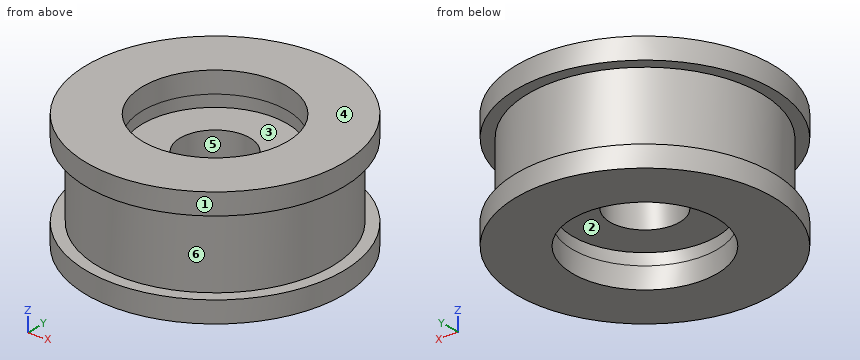
Autodesk Inventor part; units mm, degrees
ref_plane "Work Plane1" through (0, 0, 25) normal (0, 0, 1) x (1, 0, 0)
ref_plane "YZ Plane" through (0, 0, 0) normal (1, 0, 0) x (0, 1, 0)
ref_plane "XZ Plane" through (0, 0, 0) normal (0, 1, 0) x (-1, 0, 0)
sketch "Sketch1" plane through (0, 0, 0) normal (0, 0, 1) x (1, 0, 0)
  circle A0 centre (0, 0) radius 31
  circle A1 centre (0, 0) radius 55
  dimension "d0" = 62
  dimension "d1" = 110
extrude "Extrusion1" add sketch "Sketch1" along normal blind 9.12
sketch "Sketch2" plane through (0, 0, 9.12) normal (0, 0, 1) x (1, 0, 0)
  circle A0 centre (0, 0) radius 50
  circle A1 centre (0, 0) radius 15
  dimension "d4" = 100
  dimension "d5" = 30
extrude "Extrusion2" add sketch "Sketch2" along normal blind 31.76
ref_plane "Work Plane1" through (0, 0, 25) normal (0, 0, 1) x (1, 0, 0)
sketch "Sketch3" plane through (0, 0, 9.12) normal (0, 0, -1) x (-1, 0, 0)
  circle A0 centre (0, 0) radius 31
  circle A1 centre (0, 0) radius 31
  dimension "d8" = 62
extrude "Extrusion3" cut sketch "Sketch3" against normal blind 5
mirror "Mirror1" about plane through (0, 0, 25) normal (0, 0, 1) of "Extrusion1", "Extrusion3", "Extrusion2"
sketch "Sketch4" plane through (0, 0, 9.12) normal (0, 0, -1) x (-1, 0, 0)
  circle A0 centre (0, 0) radius 31
  dimension "d11" = 62
extrude "Extrusion4" cut sketch "Sketch4" against normal blind 5
properties part number "Rodillo Guia de Cadena" material "Steel, Galvanized"
The listing builds one solid part. Answer for the finished solid, in the listing's coordinates (mm). Face numbers are marked on the shaded views. A direction names the side the tool comes from. Give positions to 0.01 mm unless a question says otherwise; leave off trailing zeros. Loops run counter-clockwise (first coordinate to the right, second up) from the corner with the lowest first, then second, coordinate; pieces in that order, holes last. Notation, with made-up numbers: M 56.25,66 L 69.25,66 A23 ccw 69.25,97 Z; hole C -36,-7 d5. An arc over 180 degrees is marked long. One line per item, written item: value.
1. Find the intervals of material crossed by probe 1 along Y at (x, z) = (0, 38); probe 2 along Y at (x, z) = (0, 43.5); probe 3 along X at (y, z) = (1, 27), in increasing order.
Found:
probe 1: -50 to -31, 31 to 50
probe 2: -55 to -31, 31 to 55
probe 3: -49.99 to -14.97, 14.97 to 49.99
2. Each of these flat-tipped pins is pushed along its axis until it touches: P1, Ø3, axis at y = -18.5, z = 29.5, coming from the -X side; P2, Ø1.5, axis at x = 16, z = 37.5, coming from the -Y side; P3, Ø8, axis at y = -26, z = 20.5, coming from the +X side. Where does it stop, or does it pass through?
Found:
P1: x = -47.02
P2: y = -47.62
P3: x = 44.9
3. Section D-D on y = 28 is taken. Determine the outline of the cut face in (x, z), plus the area to 3 significant figures.
Found:
outline: M -47.34,0 L -13.3,0 L -13.3,14.12 L 13.3,14.12 L 13.3,0 L 47.34,0 L 47.34,9.12 L 41.42,9.12 L 41.42,40.88 L 47.34,40.88 L 47.34,50 L 13.3,50 L 13.3,35.88 L -13.3,35.88 L -13.3,50 L -47.34,50 L -47.34,40.88 L -41.42,40.88 L -41.42,9.12 L -47.34,9.12 Z
area: 3,610 mm^2
4. For the marked faces 1, 2 and 3, determine the directions among +Z, -Z, +X, -X, +Y, -Y from which every point of the face is accessible in a straight line to the end or side of a thin tool.
Found:
face 1: +Z, -Z
face 2: -Z
face 3: +Z
5. Section A-A on y = 0 is taken. Determine the outline of the cut face in (x, z), plus the area to 3 significant figures.
Found:
outline: M -55,0 L -31,0 L -31,14.12 L -15,14.12 L -15,35.88 L -31,35.88 L -31,50 L -55,50 L -55,40.88 L -50,40.88 L -50,9.12 L -55,9.12 Z; M 15,14.12 L 31,14.12 L 31,0 L 55,0 L 55,9.12 L 50,9.12 L 50,40.88 L 55,40.88 L 55,50 L 31,50 L 31,35.88 L 15,35.88 Z
area: 2,780 mm^2
6. Section C-C on z = 30 is taken. Determine the outline of the cut face in (x, y), plus the area to 3 significant figures.
Found:
outline: C 0,0 d100; hole C 0,0 d30
area: 7,150 mm^2
7. For a pull along Y with two mould halves and no side action, classify the marked faces 4, 5 and 6 as pulls with the +Y half, pulls with the -Y half, needs draft (parallel to the pull), parting line crosses it, or undercut.
Found:
face 4: needs draft
face 5: undercut
face 6: parting line crosses it
